```python
from build123d import *

# Parameters (mm, degrees)
SKETCH2_W                 = 25.4
SKETCH2_H                 = 25.4
SKETCH2_R                 = 1.651
BOSS_EXTRUDE1_DEPTH       = 2.8448
SKETCH3_W                 = 25.4
SKETCH3_H                 = 3.175
BOSS_EXTRUDE2_DEPTH       = 22.225
FILLET1_R                 = 2.54
F_6_CLEARANCE_HOLE1_D     = 3.7973
F_6_CLEARANCE_HOLE1_DEPTH = 12.7
F_6_CLEARANCE_HOLE1_TIP   = 1.140824014


with BuildPart() as part:
    # Sketch2 → Boss-Extrude1 (new body)
    with BuildSketch(Plane(origin=(0, 0, 0), x_dir=(1, 0, 0), z_dir=(0, 1, 0))):
        with Locations((-12.874879011, 6.594776819)):
            Rectangle(SKETCH2_W, SKETCH2_H)
        with Locations((-22.175738421, 15.230776819)):
            Circle(SKETCH2_R, mode=Mode.SUBTRACT)
        with Locations((-2.714879011, 0.879776819)):
            Circle(SKETCH2_R, mode=Mode.SUBTRACT)
    extrude(amount=BOSS_EXTRUDE1_DEPTH)

    # Sketch3 → Boss-Extrude2 (add)
    with BuildSketch(Plane(origin=(0, 0, 0), x_dir=(-1, 0, 0), z_dir=(0, -1, 0))):
        with Locations((12.874879011, -4.517723181)):
            Rectangle(SKETCH3_W, SKETCH3_H)
    extrude(amount=BOSS_EXTRUDE2_DEPTH)

    # Fillet1
    fillet1_edges = [part.edges().sort_by_distance(p)[0] for p in [
        (-12.874879011, 0, 2.930223181),
    ]]
    fillet(fillet1_edges, radius=FILLET1_R)

    # #6 Clearance Hole1
    with Locations(Plane(origin=(-6.524879011, -17.4625, 2.930223181), x_dir=(-1, 0, 0), z_dir=(0, 0, -1))):
        with Locations((0, 0), (12.7, 9.525)):
            Hole(F_6_CLEARANCE_HOLE1_D / 2, depth=F_6_CLEARANCE_HOLE1_DEPTH)
            with Locations((0, 0, -(F_6_CLEARANCE_HOLE1_DEPTH + F_6_CLEARANCE_HOLE1_TIP / 2))):  # 118° drill point
                Cone(0, F_6_CLEARANCE_HOLE1_D / 2, F_6_CLEARANCE_HOLE1_TIP, mode=Mode.SUBTRACT)


solid = part.part
```
Part model, mm, in its own coordinate system. A direction names the side the tool comes from. Round coordinates to 2 decimals unless told otherwise and drop trailing zeros. Loops run counter-clockwise (first coordinate to the right, second up) from the corner with the lowest first, then second, coordinate; pieces in that order, holes last.
1. Slice it at A-A (y = -7). Give the cut face in (x, z), and give its area (3 significant figures).
Solutions:
outline: (-25.57, 2.93) - (-20.88, 2.93) - (-20.88, 6.11) - (-25.57, 6.11) - close; (-17.57, 2.93) - (-0.17, 2.93) - (-0.17, 6.11) - (-17.57, 6.11) - close
area: 70.2 mm2
2. Slice it at B-B (x = -7.25). Give the cut face in (y, z) (3 decimals).
Solutions:
outline: (-22.225, 2.93) - (-19.217, 2.93) - (-19.217, 6.105) - (-22.225, 6.105) - close; (-15.708, 2.93) - (-2.54, 2.93) arc R2.54 cw to (0, 0.39) - (0, -19.295) - (2.845, -19.295) - (2.845, 6.105) - (-15.708, 6.105) - close
3. Two-plate mould, pull along Y, no slides. Class faces 1 (the face through (-6.77, -15.58, 4.54)), 2 (the face through (-13, 1, -19.295)), 3 (the face through (-0.928, -0.724, 2.166)), 4 (the face through (-17.414, -7.367, 4.54)): pulls with the +Y half, pulls with the -Y half, needs draft (parallel to the pull), parting line crosses it, or undercut.
Solutions:
face 1: undercut
face 2: needs draft
face 3: pulls with the -Y half
face 4: undercut
4. Slice it at D-D (x = -11). Give the cut face in (y, z) (3 decimals), and give its area (3 significant figures).
Solutions:
outline: (-22.225, 2.93) - (-2.54, 2.93) arc R2.54 cw to (0, 0.39) - (0, -19.295) - (2.845, -19.295) - (2.845, 6.105) - (-22.225, 6.105) - close
area: 144 mm2
5. Slice it at C-C (z = -14.75). Give the cut face in (x, y), and give its area (3 significant figures).
Solutions:
outline: (-25.57, 0) - (-23.76, 0) - (-23.76, 2.84) - (-25.57, 2.84) - close; (-20.6, 0) - (-0.17, 0) - (-0.17, 2.84) - (-20.6, 2.84) - close
area: 63.3 mm2
6. 3-axis set-ups, long thin cutter, end or side, ignore diameter. For faces 5 (the face through (-13, 0, -10)), 6 (the face through (-23.825, 1.402, -15.303)): which of +Z, -Z, +X, -X, +Y, -Y reach the whole face in a straight line?
Solutions:
face 5: -Z, +X, -X, -Y
face 6: +Y, -Y
7. Drill centre lines: line 1 along Z through (x, y) = (-2.75, -7.5); line 2 along Y through (x, z) = (-4.75, -12.5); line 3 along Z through (x, y) = (-11.75, -1.5). Where is each one in solid material? Low to high.
Solutions:
line 1: z = 2.93 to 6.11
line 2: y = 0 to 2.84
line 3: z = 2.71 to 6.11
8. Flat gauge pins, fed straight in: pin 1 (5 mm diameter, centred on x = -16.5, z = -2.5, fed in from -Y); pin 2 (5 mm diameter, centred on x = -19.22, y = -7.94, fed in from -Z). Where does each tip first touch, or does it go through?
Solutions:
pin 1: stops at y = 0
pin 2: stops at z = 2.93
